Here's how the part is built. I have some questions about the finished solid (model axes, mm). Round coordinates to 2 decimals unless told otherwise and drop trailing zeros. Order: outer loops, then holes, each group sorted by start corner. A loop starts at its lowest first (then second) coordinate and runs counter-clockwise, first axis right, second up.
```python
from build123d import *

# Parameters (mm, degrees)
BOSS_EXTRUDE1_DEPTH = 120


with BuildPart() as part:
    # Sketch1 → Boss-Extrude1 (new body)
    with BuildSketch(Plane(origin=(0, 0, 0), x_dir=(1, 0, 0), z_dir=(0, 1, 0))):
        with BuildLine():
            Line((-3, 0), (-3, -1.6))
            Line((-3, -1.6), (-4, -1.6))
            Line((-4, -1.6), (-2.599584924, -3.6))
            Line((-2.599584924, -3.6), (2.599584924, -3.6))
            Line((2.599584924, -3.6), (4, -1.6))
            Line((4, -1.6), (3, -1.6))
            Line((3, -1.6), (3, 0))
            Line((3, 0), (48, 0))
            Line((48, 0), (48, 0.8))
            Line((48, 0.8), (-23, 0.8))
            ThreePointArc((-23, 0.8), (-153.089844763, -122.665428697), (-187.317261189, -298.720998783))
            Line((-187.317261189, -298.720998783), (-186.319141297, -297.948173118))
            ThreePointArc((-186.319141297, -297.948173118), (-152.080290875, -122.980601765), (-23, 0))
            Line((-23, 0), (-3, 0))
        make_face()
    extrude(amount=BOSS_EXTRUDE1_DEPTH)


solid = part.part
```
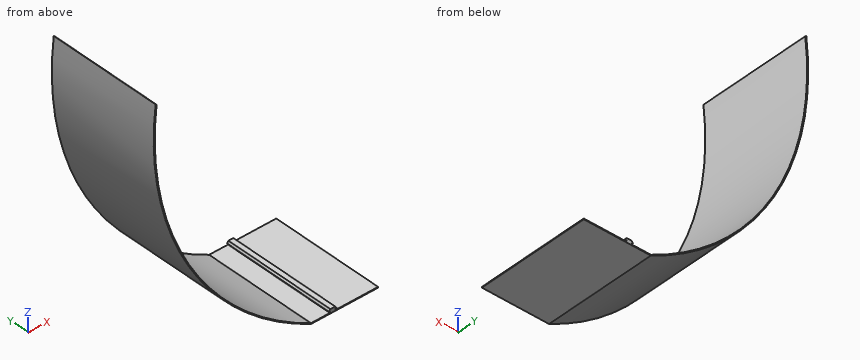
1. I'm going to push flat-ended pins straight in: P1, Ø8, axis at x = -76, y = 68, coming from the -Z side; P2, Ø10, axis at x = -11.5, y = 74, coming from the +Z side; P3, Ø12, axis at y = 82, z = 142.5, coming from the +X side. Where does each tip first touch, or does it pass through?
Evaluation:
P1: stops at z = 29.05
P2: stops at z = 0
P3: stops at x = -159.04
2. If we section it at A-A, the plane y = 27.5: Write out the boundary of the cut face in (x, z).
Evaluation:
outline: (-187.32, 298.72) arc R294.19 ccw to (-23, -0.8) - (48, -0.8) - (48, 0) - (3, 0) - (3, 1.6) - (4, 1.6) - (2.6, 3.6) - (-2.6, 3.6) - (-4, 1.6) - (-3, 1.6) - (-3, 0) - (-23, 0) arc R293.89 cw to (-186.32, 297.95) - close
3. I need wall thicknesses on probe 1 along Z at (x, y) = (32, 108); probe 2 along X at (y, z) = (11, 48.5); probe 3 along X at (y, z) = (99, 222). Which ranges of each line are inside material? Lowest first, please.
Evaluation:
probe 1: z = -0.8 to 0
probe 2: x = -95.26 to -93.93
probe 3: x = -186.32 to -185.21
4. If we section it at C-C, the plane z = 164.5: Write out the boundary of the cut face in (x, y), and give its area (3 significant figures).
Evaluation:
outline: (-171.96, 0) - (-170.81, 0) - (-170.81, 120) - (-171.96, 120) - close
area: 137 mm2
5. If we section it at B-B, the plane x = 33: Write out the boundary of the cut face in (y, z).
Evaluation:
outline: (0, -0.8) - (120, -0.8) - (120, 0) - (0, 0) - close
